```python
from build123d import *

# Parameters (mm, degrees)
BOSS_EXTRUDE1_DEPTH = 12.7
CUT_EXTRUDE1_DEPTH  = 164.974925036
SKETCH3_R           = 2.5
CUT_EXTRUDE2_DEPTH  = 164.974925036


with BuildPart() as part:
    # Sketch1 → Boss-Extrude1 (new body)
    with BuildSketch(Plane.XY):
        with BuildLine():
            Line((-60.262418021, -86.089619685), (122.036781237, -86.089619685))
            Line((122.036781237, -86.089619685), (122.036781237, 96.209579573))
            Line((122.036781237, 96.209579573), (109.464422667, 108.781938142))
            Line((109.464422667, 108.781938142), (95.096012874, 94.413528349))
            ThreePointArc((95.096012874, 94.413528349), (8.18551326, 27.761648291), (-58.466366797, -59.148851322))
            Line((-58.466366797, -59.148851322), (-72.83477659, -73.517261115))
            Line((-72.83477659, -73.517261115), (-60.262418021, -86.089619685))
        make_face()
    extrude(amount=BOSS_EXTRUDE1_DEPTH)

    # Sketch2 → Cut-Extrude1 (cut, through all)
    with BuildSketch(Plane.XY.offset(12.7)):
        with BuildLine():
            Line((96.548355206, 57.447236553), (102.693314786, -59.805577132))
            ThreePointArc((102.693314786, -59.805577132), (100.768098522, -64.82093697), (95.752738684, -66.746153234))
            Line((95.752738684, -66.746153234), (-21.500075001, -60.601193655))
            ThreePointArc((-21.500075001, -60.601193655), (-27.048234767, -56.985522244), (-26.669858487, -50.374018034))
            ThreePointArc((-26.669858487, -50.374018034), (24.070759008, 11.876402544), (86.321179585, 62.617020039))
            ThreePointArc((86.321179585, 62.617020039), (92.932683796, 62.995396319), (96.548355206, 57.447236553))
        make_face()
    extrude(amount=-CUT_EXTRUDE1_DEPTH, mode=Mode.SUBTRACT)

    # Sketch3 → Cut-Extrude2 (cut, through all)
    with BuildSketch(Plane(origin=(0, 0, 0), x_dir=(-1, 0, 0), z_dir=(0, 0, -1))):
        with Locations((-100.449569709, 56.599670194)):
            Circle(SKETCH3_R)
        with Locations((-79.287603593, 63.568690871)):
            Circle(SKETCH3_R)
        with Locations((-39.228116315, 32.54613876)):
            Circle(SKETCH3_R)
        with Locations((-3.401022792, -3.280954763)):
            Circle(SKETCH3_R)
        with Locations((27.621529319, -43.340442042)):
            Circle(SKETCH3_R)
        with Locations((20.652508642, -64.502408157)):
            Circle(SKETCH3_R)
        with Locations((-35.508445898, -67.856108518)):
            Circle(SKETCH3_R)
        with Locations((-91.669400439, -71.209808879)):
            Circle(SKETCH3_R)
        with Locations((-107.156970431, -55.722238887)):
            Circle(SKETCH3_R)
        with Locations((-103.80327007, 0.438715653)):
            Circle(SKETCH3_R)
    extrude(amount=-CUT_EXTRUDE2_DEPTH, mode=Mode.SUBTRACT)


solid = part.part
```
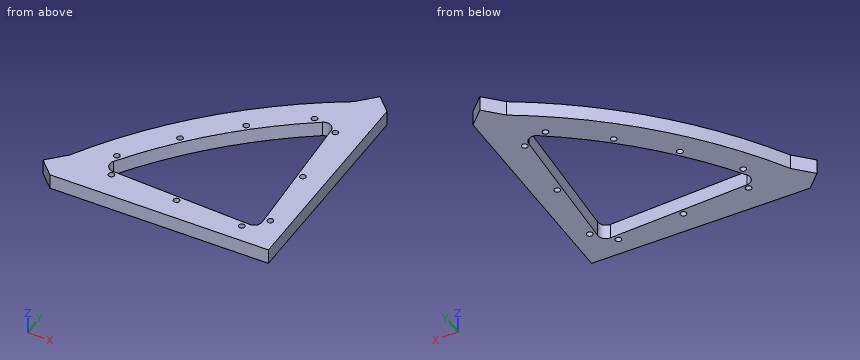
Can you work these out from the model? Positions are in its coordinate system, mm. Coordinates: 2 decimals unless noted, no trailing zeros. Loops run counter-clockwise (first coordinate to the right, second up) from the corner with the lowest first, then second, coordinate; pieces in that order, holes last.
Item 1: Suppose I cut it at B-B (y = -11.5). Please give me the cut outline in (x, z), then the cut area to 3 significant figures.
Answers below:
outline: (-26.45, 0) - (2.5, 0) - (2.5, 12.7) - (-26.45, 12.7) - close; (100.16, 0) - (122.04, 0) - (122.04, 12.7) - (100.16, 12.7) - close
area: 645 mm2
Item 2: Suppose I cut it at D-D (x = -33.5). Please give me the cut outline in (y, z), then the cut area to 3 significant figures.
Answers below:
outline: (-86.09, 0) - (-20.85, 0) - (-20.85, 12.7) - (-86.09, 12.7) - close
area: 829 mm2
Item 3: I'm going to push flat-ended pins straight in: pin 1 (6.5 mm diameter, centred on x = 3.4, y = -3.28, fed in from +Z); pin 2 (5 mm diameter, centred on x = 49, z = 7.5, fed in from +Y). Where does each tip first touch, or does it pass through?
Answers below:
pin 1: stops at z = 12.7
pin 2: stops at y = 65.5
Item 4: Suppose I cut it at A-A (x = 53). Please give me the cut outline in (y, z).
Answers below:
outline: (-86.09, 0) - (-64.51, 0) - (-64.51, 12.7) - (-86.09, 12.7) - close; (38.09, 0) - (66.63, 0) - (66.63, 12.7) - (38.09, 12.7) - close
Item 5: Suppose I cut it at C-C (z = 4). State how many separate pieces and enclosed holes the cut face has, then the cut area to 3 significant figures.
Answers below:
separate pieces: 1
enclosed holes: 11
area: 12,700 mm2
Item 6: Please list where these lines run through material, in increasing order: L1, parallel to X at y = 33.5, z = 6.75; L2, parallel to Y at x = 80, z = 7; L3, parallel to X at y = -56.5, z = 2.25.
Answers below:
L1: x = 14.04 to 36.92, 41.54 to 47.51, 97.8 to 122.04
L2: y = -86.09 to -65.92, 58.37 to 61.17, 65.97 to 85.28
L3: x = -56.93 to -27.27, 102.52 to 104.78, 109.53 to 122.04
